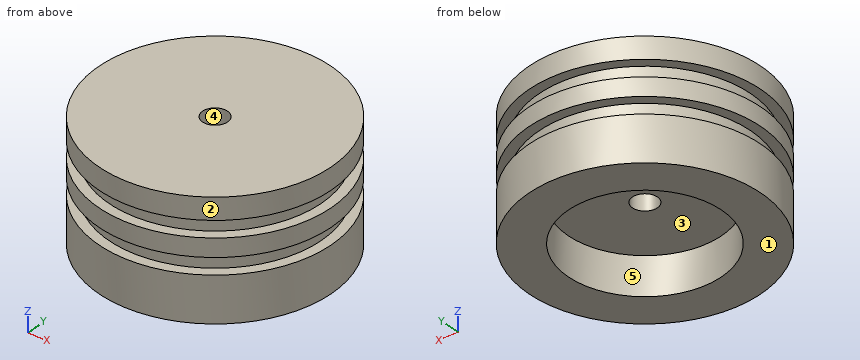
```python
from build123d import *

# Parameters (mm, degrees)
F0_R      = 16.256
F1_DEPTH  = 6.35
F2_R      = 14.859
F3_DEPTH  = 16.002
F5_R      = 16.256
F6_DEPTH  = 2.54
F8_R      = 16.256
F9_DEPTH  = 3.0226
F10_R     = 1.75
F11_DEPTH = 42.672
F12_R     = 1.75
F13_DEPTH = 37.084
F14_R     = 10.75
F15_DEPTH = 5.334


with BuildPart() as f1:
    # F0 (on Top) → F1 (new body)
    with BuildSketch(Plane.XY):
        Circle(F0_R)
    extrude(amount=F1_DEPTH)

    # F2 (on Top) → F3 (join)
    with BuildSketch(Plane.XY):
        Circle(F2_R)
    extrude(amount=F3_DEPTH)

    # F5 (on offset) → F6 (join)
    with BuildSketch(Plane.XY.offset(8.636)):
        Circle(F5_R)
    extrude(amount=F6_DEPTH)

    # F8 (on offset) → F9 (join)
    with BuildSketch(Plane.XY.offset(13.462)):
        Circle(F8_R)
    extrude(amount=F9_DEPTH)

    # F10 (on offset) → F11 (cut)
    with BuildSketch(Plane.XY.offset(13.462)):
        Circle(F10_R)
    extrude(amount=F11_DEPTH, mode=Mode.SUBTRACT)

    # F12 (on Top) → F13 (cut)
    with BuildSketch(Plane.XY):
        Circle(F12_R)
    extrude(amount=F13_DEPTH, mode=Mode.SUBTRACT)

    # F14 (on Top) → F15 (cut)
    with BuildSketch(Plane.XY):
        Circle(F14_R)
    extrude(amount=F15_DEPTH, mode=Mode.SUBTRACT)


solid = f1.part
```
Can you work these out from the model? Positions are in its coordinate system, mm. Face numbers are marked on the shaded views. A direction names the side the tool comes from. Coordinates: 2 decimals unless noted, no trailing zeros. Loops run counter-clockwise (first coordinate to the right, second up) from the corner with the lowest first, then second, coordinate; pieces in that order, holes last. Notation, with made-up numbers: (-21, -30) -> (-7, -30) arc R8 ccw to (-7, -19) -> close; hole circle Ø5 at (20.5, -18.5). An arc over 180 degrees is marked (long way). Put each result on its own line as item: value. Start each with the question number.
Q1. If I drill on line 1 (Y direction, x = 0, z = 9.5); line 2 (X direction, y = 0, z = 12); line 3 (Y direction, x = 0, z = 1.2), over which ranges is the centre line in solid material (lowest first)? Write a range as [from, to].
Q2. I want a section at A-A (y = 0). Write out the boundary of the cut face in (x, z).
Q3. I want a section at D-D (x = 13). Write out the boundary of the cut face in (y, z).
Q4. For the marked faces 4 and 5, which set-ups out of +Z, -Z, +X, -X, +Y, -Y let a thin tool reach every point of the face, with its end or its side?
Q5. I'm going to push flat-ended pins straight in: P1, Ø2, axis at y = -9.5, z = 7.5, coming from the -X side; P2, Ø1.5, axis at x = 3, z = 5.5, coming from the -Y side; P3, Ø1, axis at y = -4, z = 7.5, coming from the +X side; P4, Ø3, axis at x = 0, y = 0, coming from the +Z side. Where does each tip first touch, or does it pass through?
Q6. I want a section at C-C (z = 10). Write out the boundary of the cut face in (x, y).
Q7. Thinking about a two-plate mould opening in X: for the marked faces 1, 2 and 3, which applies, pulls with the +X half, pulls with the -X half, needs draft (parallel to the pull), parting line crosses it, or undercut?
Taken from the geometry:
1. line 1: y = [-16.26, -1.75], [1.75, 16.26]
1. line 2: x = [-14.86, -1.75], [1.75, 14.86]
1. line 3: y = [-16.26, -10.75], [10.75, 16.26]
2. outline: (-16.26, 0) -> (-10.75, 0) -> (-10.75, 5.33) -> (-1.75, 5.33) -> (-1.75, 16.48) -> (-16.26, 16.48) -> (-16.26, 13.46) -> (-14.86, 13.46) -> (-14.86, 11.18) -> (-16.26, 11.18) -> (-16.26, 8.64) -> (-14.86, 8.64) -> (-14.86, 6.35) -> (-16.26, 6.35) -> close; (1.75, 5.33) -> (10.75, 5.33) -> (10.75, 0) -> (16.26, 0) -> (16.26, 6.35) -> (14.86, 6.35) -> (14.86, 8.64) -> (16.26, 8.64) -> (16.26, 11.18) -> (14.86, 11.18) -> (14.86, 13.46) -> (16.26, 13.46) -> (16.26, 16.48) -> (1.75, 16.48) -> close
3. outline: (-9.76, 0) -> (9.76, 0) -> (9.76, 6.35) -> (7.2, 6.35) -> (7.2, 8.64) -> (9.76, 8.64) -> (9.76, 11.18) -> (7.2, 11.18) -> (7.2, 13.46) -> (9.76, 13.46) -> (9.76, 16.48) -> (-9.76, 16.48) -> (-9.76, 13.46) -> (-7.2, 13.46) -> (-7.2, 11.18) -> (-9.76, 11.18) -> (-9.76, 8.64) -> (-7.2, 8.64) -> (-7.2, 6.35) -> (-9.76, 6.35) -> close
4. face 4: +Z, -Z
4. face 5: -Z
5. P1: stops at x = -12.19
5. P2: stops at y = -16.1
5. P3: stops at x = 14.44
5. P4: passes through
6. outline: circle Ø32.51 at (0, 0); hole circle Ø3.5 at (0, 0)
7. face 1: needs draft
7. face 2: parting line crosses it
7. face 3: undercut
